The figure shows three views and two pictorial views of one solid part (mm, origin at its lowest corner). Answer the questions. Round coordinates to 2 decimals unless told otherwise and drop trailing zeros. Order: outer loops, then holes, each group sorted by start corner. A loop starts at its lowest first (then second) coordinate and runs counter-clockwise, first axis right, second up. Notation, with made-up numbers: M 85.5,32 L 129.5,32 A32 cw 129.5,59 Z; hole C 3.5,-10.75 d3. An arc over 180 degrees is marked long. Answer as CSV lines item,"result".
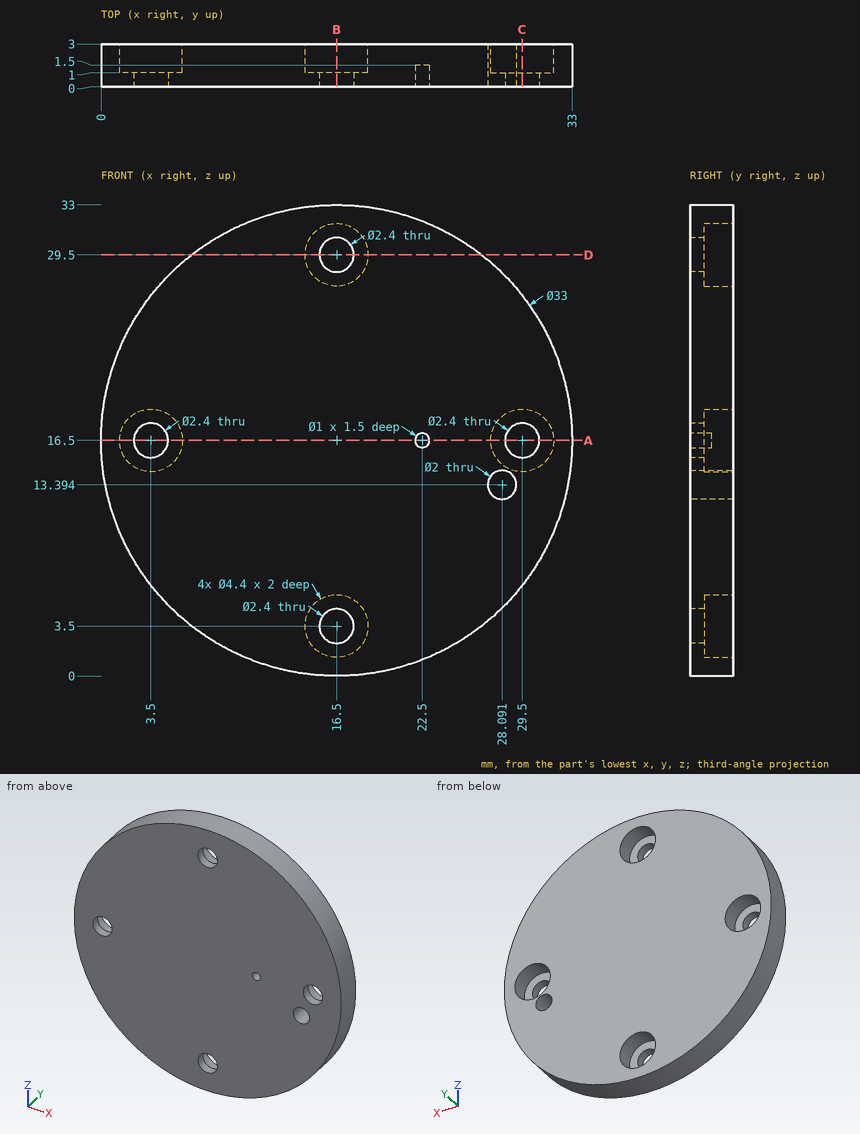
Item 1: A cutting plane is placed at C-C, the plane x = 29.5. Determine the outline of the cut face in (y, z), and give its area (3 significant figures).
Ans:
outline,"M 0,6.34 L 3,6.34 L 3,14.3 L 1,14.3 L 1,15.3 L 0,15.3 Z; M 0,17.7 L 1,17.7 L 1,18.7 L 3,18.7 L 3,26.66 L 0,26.66 Z"
area,"49.8 mm2"
Item 2: Flat-ended cylindrical pins translate along their axes: pin 1 (1.5 mm diameter, centred on y = 0.5, z = 13.5, fed in from -X); pin 2 (2.5 mm diameter, centred on x = 3.5, z = 16.5, fed in from -Y); pin 3 (1.5 mm diameter, centred on x = 22.5, y = 1.5, fed in from +Z); pin 4 (2.5 mm diameter, centred on x = 16.5, z = 3.5, fed in from +Y). Find the tip coordinate at first contact, or state that the pin passes through.
Ans:
pin 1,"x = 0.15"
pin 2,"y = 0"
pin 3,"z = 32.14"
pin 4,"y = 1"
Item 3: A cutting plane is placed at B-B, the plane x = 16.5. Determine the outline of the cut face in (y, z), and give its area (3 significant figures).
Ans:
outline,"M 0,0 L 3,0 L 3,1.3 L 1,1.3 L 1,2.3 L 0,2.3 Z; M 0,4.7 L 1,4.7 L 1,5.7 L 3,5.7 L 3,27.3 L 1,27.3 L 1,28.3 L 0,28.3 Z; M 0,30.7 L 1,30.7 L 1,31.7 L 3,31.7 L 3,33 L 0,33 Z"
area,"76.6 mm2"
Item 4: A cutting plane is placed at A-A, the plane z = 16.5. Determine the outline of the cut face in (x, y).
Ans:
outline,"M 0,0 L 2.3,0 L 2.3,1 L 1.3,1 L 1.3,3 L 0,3 Z; M 4.7,0 L 22,0 L 22,1.5 L 23,1.5 L 23,0 L 28.3,0 L 28.3,1 L 27.3,1 L 27.3,3 L 5.7,3 L 5.7,1 L 4.7,1 Z; M 30.7,0 L 33,0 L 33,3 L 31.7,3 L 31.7,1 L 30.7,1 Z"
Item 5: A cutting plane is placed at D-D, the plane z = 29.5. Determine the outline of the cut face in (x, y), and give its area (3 significant figures).
Ans:
outline,"M 6.34,0 L 15.3,0 L 15.3,1 L 14.3,1 L 14.3,3 L 6.34,3 Z; M 17.7,0 L 26.66,0 L 26.66,3 L 18.7,3 L 18.7,1 L 17.7,1 Z"
area,"49.8 mm2"
Item 6: Find the intervals of material crossed by probe 1 along Z at (x, y) = (17, 2.15); probe 2 along Y at (x, z) = (18, 4); probe 3 along X at (y, z) = (0.65, 3.5), in increasing order. Write a range as [from, to].
Ans:
probe 1,"[0.01, 1.36], [5.64, 27.36], [31.64, 32.99]"
probe 2,"[0, 1]"
probe 3,"[6.34, 15.3], [17.7, 26.66]"
